Check sheet for the drawn part. Datum: minimum x, y, z corner. Units: mm. Coordinates: 2 decimals unless noted, no trailing zeros. Loops run counter-clockwise (first coordinate to the right, second up) from the corner with the lowest first, then second, coordinate; pieces in that order, holes last. Notation, with made-up numbers: (61, -24) -> (71, -24) arc R30 ccw to (71, 3) -> close; hole circle Ø5 at (-37, 35.25). An arc over 180 degrees is marked (long way). Use CSV: the item, a comma, the result in double quotes. Start each with the question number.
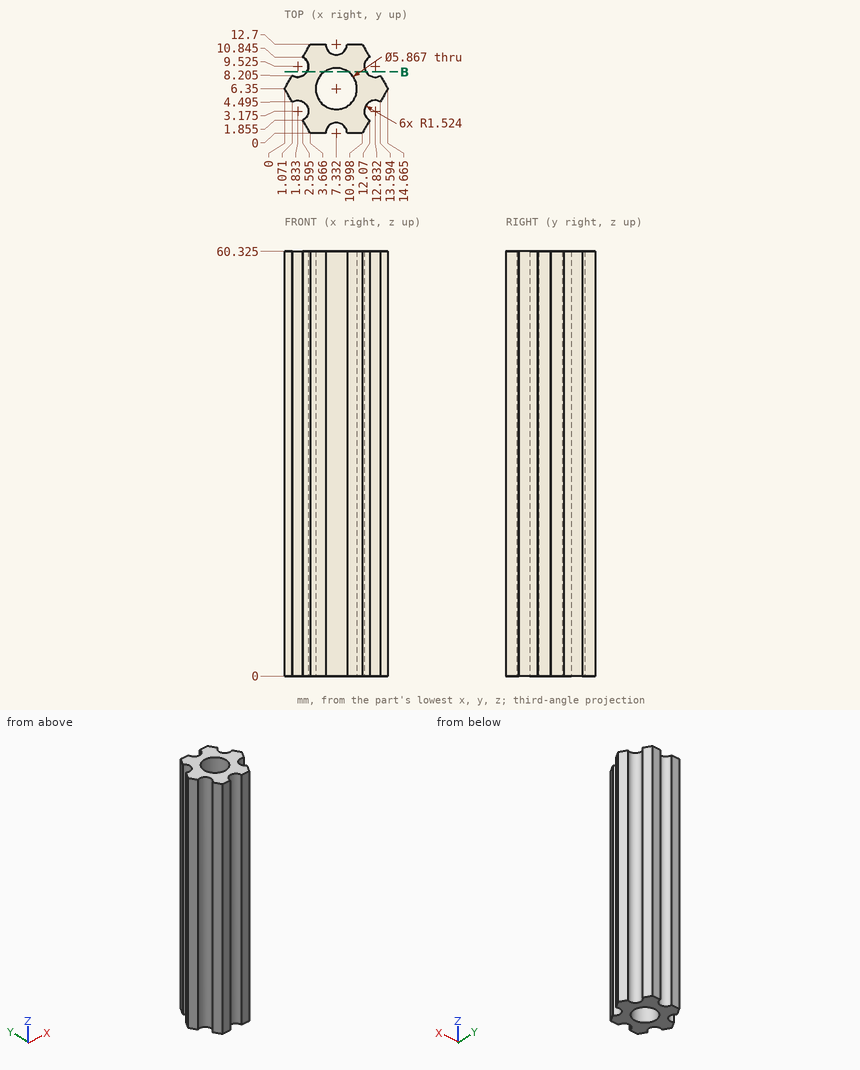
1. Depth check by flat-ended pin: pin 1 (6 mm diameter, centred on x = 12.5, z = 50.5, fed in from +Y). Enter the tip coordinate at first touch or a pass-through.
2. Scan lines: line 1 (Y direction, x = 11.5, z = 19) (1 decimal); line 2 (Y direction, x = 2.75, z = 33) (1 decimal); line 3 (Y direction, x = 9, z = 44) (1 decimal). Record each from-to range of solid material in increasing order.
3. Cross-section at B-B, the plane y = 8.75. Record the boundary of the cut face in (x, z) (1 decimal).
Solution:
1,pin 1,"stops at y = 12.7"
2,line 1,"y = 0.9 to 2.4, 3.9 to 8.8, 10.3 to 11.8"
2,line 2,"y = 1.6 to 2, 4.4 to 8.3, 10.7 to 11.1"
2,line 3,"y = 0 to 3.9, 8.8 to 12.7"
3,outline,"(3.1, 0) -> (5.6, 0) -> (5.6, 60.3) -> (3.1, 60.3) -> close; (9, 0) -> (11.5, 0) -> (11.5, 60.3) -> (9, 60.3) -> close"
